```python
from build123d import *

# Parameters (mm, degrees)
ESTRUSIONE_ESTRUSIONE1_DEPTH = 60
RACCORDO1_R                  = 1
RACCORDO2_R                  = 1
TAGLIO_ESTRUSIONE1_REACH     = 116.198
SCHIZZO2_R                   = 1.75
SCHIZZO2_R_2                 = 3
SCHIZZO3_R                   = 3.5
TAGLIO_ESTRUSIONE2_DEPTH     = 115.494541355


with BuildPart() as part:
    # Schizzo1 → Estrusione-Estrusione1 (new body)
    with BuildSketch(Plane.XY):
        Polygon((-95, 22), (-95, 0), (0, 0), (0, 1.6), (-93.4, 1.6), (-93.4, 22), align=None)
    extrude(amount=ESTRUSIONE_ESTRUSIONE1_DEPTH)

    # Raccordo1
    raccordo1_edges = [part.edges().sort_by_distance(p)[0] for p in [
        (-95, 0, 30),
    ]]
    fillet(raccordo1_edges, radius=RACCORDO1_R)

    # Raccordo2
    raccordo2_edges = [part.edges().sort_by_distance(p)[0] for p in [
        (-93.4, 1.6, 30),
    ]]
    fillet(raccordo2_edges, radius=RACCORDO2_R)

    # Schizzo2 → Taglio-Estrusione1 (cut, up to next)
    with BuildSketch(Plane(origin=(0, 1.6, 0), x_dir=(1, 0, 0), z_dir=(0, 1, 0)), mode=Mode.PRIVATE) as taglio_estrusione1_sk1:
        with Locations(Location((-31, -5, 0), (0, 0, 180))):
            Circle(SCHIZZO2_R)
    taglio_estrusione1_tool1 = extrude(taglio_estrusione1_sk1.sketch, amount=-TAGLIO_ESTRUSIONE1_REACH, mode=Mode.PRIVATE) & part.part
    # Schizzo2 → Taglio-Estrusione1 (cut, up to next)
    with BuildSketch(Plane(origin=(0, 1.6, 0), x_dir=(1, 0, 0), z_dir=(0, 1, 0)), mode=Mode.PRIVATE) as taglio_estrusione1_sk2:
        with Locations(Location((-31, -30, 0), (0, 0, 180))):
            Circle(SCHIZZO2_R_2)
    taglio_estrusione1_tool2 = extrude(taglio_estrusione1_sk2.sketch, amount=-TAGLIO_ESTRUSIONE1_REACH, mode=Mode.PRIVATE) & part.part
    # Schizzo2 → Taglio-Estrusione1 (cut, up to next)
    with BuildSketch(Plane(origin=(0, 1.6, 0), x_dir=(1, 0, 0), z_dir=(0, 1, 0)), mode=Mode.PRIVATE) as taglio_estrusione1_sk3:
        with Locations(Location((-31, -55, 0), (0, 0, 180))):
            Circle(SCHIZZO2_R)
    taglio_estrusione1_tool3 = extrude(taglio_estrusione1_sk3.sketch, amount=-TAGLIO_ESTRUSIONE1_REACH, mode=Mode.PRIVATE) & part.part
    add(taglio_estrusione1_tool1.solids().sort_by_distance((-31, 1.6, 5))[0], mode=Mode.SUBTRACT)
    add(taglio_estrusione1_tool2.solids().sort_by_distance((-31, 1.6, 30))[0], mode=Mode.SUBTRACT)
    add(taglio_estrusione1_tool3.solids().sort_by_distance((-31, 1.6, 55))[0], mode=Mode.SUBTRACT)

    # Schizzo3 → Taglio-Estrusione2 (cut, through all)
    with BuildSketch(Plane.ZY.offset(95)):
        with Locations((11.5, 11)):
            Circle(SCHIZZO3_R)
        with Locations((48.5, 11)):
            Circle(SCHIZZO3_R)
    extrude(amount=-TAGLIO_ESTRUSIONE2_DEPTH, mode=Mode.SUBTRACT)


solid = part.part
```
Work out the finished part from the listing and answer in its coordinate system (mm). A direction names the side the tool comes from. Give positions to 0.01 mm unless a question says otherwise; leave off trailing zeros. Order: outer loops, then holes, each group sorted by start corner. A loop starts at its lowest first (then second) coordinate and runs counter-clockwise, first axis right, second up.
1. Section B-B, the plane y = 11 is taken. Determine the outline of the cut face in (x, z), and give its area (3 significant figures).
Result sheet:
outline: (-95, 0) - (-93.4, 0) - (-93.4, 8) - (-95, 8) - close; (-95, 15) - (-93.4, 15) - (-93.4, 45) - (-95, 45) - close; (-95, 52) - (-93.4, 52) - (-93.4, 60) - (-95, 60) - close
area: 73.6 mm2
2. Each of these flat-tipped pins is pushed along its axis until it touches: P1, Ø18, axis at x = -52.5, z = 17, coming from the +Y side; P2, Ø4, axis at y = 11, z = 11.5, coming from the +X side; P3, Ø11, axis at y = 11, z = 48.5, coming from the +X side. Where does it stop, or does it pass through?
Result sheet:
P1: stops at y = 1.6
P2: passes through
P3: stops at x = -93.4
3. The mould has two halves that part along Z. Classify faces 1 (the cylindrical face through (-29.25, 0.81, 5.08)), 2 (the flat face through (-48, 0, 30)), 3 (the flat face through (-62, 1, 0)), 4 (the flat face through (-62, 1, 60)): released by +Z, released by -Z, zero draft, split by the parting line, or undercut.
Result sheet:
face 1: undercut
face 2: zero draft
face 3: released by -Z
face 4: released by +Z
4. Section D-D, the plane x = -40 is taken. Determine the outline of the cut face in (y, z), and give its area (3 significant figures).
Result sheet:
outline: (0, 0) - (1.6, 0) - (1.6, 60) - (0, 60) - close
area: 96.0 mm2
5. For faces 5 (the cylindrical face through (-94.211, 7.583, 10.741)), 6 (the flat face through (-46, 1.6, 30)), determine the directions among +Z, -Z, +X, -X, +Y, -Y from which every point of the face is accessible in a straight line to the end or side of a thin tool.
Result sheet:
face 5: +X, -X
face 6: +Z, -Z, +X, +Y
6. Section A-A, the plane z = 55 is taken. Determine the outline of the cut face in (x, y).
Result sheet:
outline: (-95, 1) arc R1 ccw to (-94, 0) - (-32.75, 0) - (-32.75, 1.6) - (-92.4, 1.6) arc R1 cw to (-93.4, 2.6) - (-93.4, 22) - (-95, 22) - close; (-29.25, 0) - (0, 0) - (0, 1.6) - (-29.25, 1.6) - close
7. Straight lines are drawn through the part: L1, parallel to Z at x = -31, y = 0.8; L2, parallel to Y at x = -72, z = 33.5; L3, parallel to X at y = 20.75, z = 51.5. For each, find the intervals that lie inside material, in ascending order.
Result sheet:
L1: z = 0 to 3.25, 6.75 to 27, 33 to 53.25, 56.75 to 60
L2: y = 0 to 1.6
L3: x = -95 to -93.4
8. Section C-C, the plane z = 43 is taken. Determine the outline of the cut face in (x, y).
Result sheet:
outline: (-95, 1) arc R1 ccw to (-94, 0) - (0, 0) - (0, 1.6) - (-92.4, 1.6) arc R1 cw to (-93.4, 2.6) - (-93.4, 22) - (-95, 22) - close
